```python
from build123d import *

# Parameters (mm, degrees)
ESBO_O1_R                = 4
ESBO_O1_R_2              = 1.85
ESBO_O1_W                = 8
ESBO_O1_H                = 8
RESSALTO_EXTRUS_O1_DEPTH = 10
FILETE1_R                = 20


with BuildPart() as part:
    # Esboço1 → Ressalto-extrusão1 (new body)
    with BuildSketch(Plane.XY):
        with BuildLine():
            Line((80.144957554, -18.086974533), (50, 0))
            Line((50, 0), (0, 0))
            Line((0, 0), (-50, 0))
            Line((-50, 0), (-80.144957554, -18.086974533))
            ThreePointArc((-80.144957554, -18.086974533), (-83.574929257, -31.806861344), (-69.855042446, -35.236833047))
            Line((-69.855042446, -35.236833047), (-50, -23.323807579))
            Line((-50, -23.323807579), (50, -23.323807579))
            Line((50, -23.323807579), (69.855042446, -35.236833047))
            ThreePointArc((69.855042446, -35.236833047), (83.574929257, -31.806861344), (80.144957554, -18.086974533))
        make_face()
        with Locations((-50, -11.66190379)):
            Circle(ESBO_O1_R, mode=Mode.SUBTRACT)
        with Locations(Location((50, -11.66190379, 0), (0, 0, 180))):
            Circle(ESBO_O1_R, mode=Mode.SUBTRACT)
        with Locations((0, -11.66190379)):
            Circle(ESBO_O1_R_2, mode=Mode.SUBTRACT)
        with Locations((-75, -26.66190379)):
            Circle(ESBO_O1_R, mode=Mode.SUBTRACT)
        with Locations(Location((75, -26.66190379, 0), (0, 0, 180))):
            Circle(ESBO_O1_R, mode=Mode.SUBTRACT)
        with Locations((20, -11.66190379)):
            Rectangle(ESBO_O1_W, ESBO_O1_H, mode=Mode.SUBTRACT)
        with Locations((-20, -11.66190379)):
            Rectangle(ESBO_O1_W, ESBO_O1_H, mode=Mode.SUBTRACT)
    extrude(amount=RESSALTO_EXTRUS_O1_DEPTH)

    # Filete1
    filete1_edges = [part.edges().sort_by_distance(p)[0] for p in [
        (-50, 0, 5),
        (50, 0, 5),
    ]]
    fillet(filete1_edges, radius=FILETE1_R)


solid = part.part
```
Read the model definition and answer for the solid it produces. Units are mm, in the model's axes. A direction names the side the tool comes from. Coordinates: 2 decimals unless noted, no trailing zeros. Write each loop counter-clockwise with the first axis right and the second up, starting at its lowest first coordinate (ties: lowest second). Pieces come first, ordered by that corner, then holes. Notation, with made-up numbers: (-31, -13.75) -> (-26, -13.75) arc R32 ccw to (-26, 16.25) -> close; hole circle Ø8 at (-8, 63). An arc over 180 degrees is marked (long way). Write item = value, one per line.
(1) Section A-A on x = -75 is taken. Write down the section's boundary in (y, z), plus the area to 3 significant figures.
From the geometry:
outline = (-36.66, 0) -> (-30.66, 0) -> (-30.66, 10) -> (-36.66, 10) -> close; (-22.66, 0) -> (-15, 0) -> (-15, 10) -> (-22.66, 10) -> close
area = 137 mm2
(2) For a pull along Z with two mould halves and no side action, classify faces 4 (the face through (83.46, -31.99, 4.93)), 5 (the face through (-1, -14, 0)) as +Z half, -Z half, draft (parallel to the pull), parting line (faces both ways), or undercut.
From the geometry:
face_4 = draft
face_5 = -Z half
(3) Section B-B on z = 7 is taken. Write down the section's boundary in (x, y).
From the geometry:
outline = (-80.14, -18.09) arc R10 ccw to (-69.86, -35.24) -> (-50, -23.32) -> (50, -23.32) -> (69.86, -35.24) arc R10 ccw to (80.14, -18.09) -> (54.75, -2.85) arc R20 ccw to (44.46, 0) -> (-44.46, 0) arc R20 ccw to (-54.75, -2.85) -> close; hole circle Ø8 at (-75, -26.66); hole circle Ø8 at (-50, -11.66); hole (-24, -15.66) -> (-16, -15.66) -> (-16, -7.66) -> (-24, -7.66) -> close; hole circle Ø3.7 at (0, -11.66); hole (16, -15.66) -> (24, -15.66) -> (24, -7.66) -> (16, -7.66) -> close; hole circle Ø8 at (50, -11.66); hole circle Ø8 at (75, -26.66)
(4) Section C-C on x = 0 is taken. Write down the section's boundary in (y, z).
From the geometry:
outline = (-23.32, 0) -> (-13.51, 0) -> (-13.51, 10) -> (-23.32, 10) -> close; (-9.81, 0) -> (0, 0) -> (0, 10) -> (-9.81, 10) -> close
(5) Section D-D on y = -5.5 is taken. Write down the section's boundary in (x, z).
From the geometry:
outline = (-59.17, 0) -> (59.17, 0) -> (59.17, 10) -> (-59.17, 10) -> close
(6) Given pin 1 Ø2.5 at (y, z) = (-11, 6) entering from -X; pin 2 Ø5 at (y, z) = (-6, 4.5) entering from -X; pin 3 Ø6.5 at (x, y) = (-50, -11.66) entering from -Z; pin 4 Ø2.5 at (x, z) = (-19, 6.5) entering from -Y, each flat-ended and moving along its own axis, determine where each tip first touches the part or whether it passes through.
From the geometry:
pin_1 = -70.42
pin_2 = -64.17
pin_3 = through
pin_4 = -23.32
(7) Which of the six approach directions +Z, -Z, +X, -X, +Y, -Y give full straight-line access (tool end or side, diameter ignored) to faces 1 (the face through (59.79, -29.2, 4.93)), 2 (the face through (16, -12, 5)), 3 (the face through (67.63, -10.58, 4.93))?
From the geometry:
face_1 = +Z, -Z, -Y
face_2 = +Z, -Z
face_3 = +Z, -Z, +X, +Y
(8) Straight lines are drawn through the part: L1, parallel to Y at x = 0, z = 5.75; L2, parallel to X at y = -11, z = 6.25; L3, parallel to X at y = -8, z = 7.75. For each, find the intervals that lie inside material, in ascending order. Write a range as from..to.
From the geometry:
L1 = -23.32..-13.51, -9.81..0
L2 = -68.33..-53.94, -46.06..-24, -16..-1.73, 1.73..16, 24..46.06, 53.94..68.33
L3 = -63.33..-51.61, -48.39..-24, -16..16, 24..48.39, 51.61..63.33
